Verification items for the finished model (mm, model axes). Round coordinates to 2 decimals unless told otherwise and drop trailing zeros. Write each loop counter-clockwise with the first axis right and the second up, starting at its lowest first coordinate (ties: lowest second). Pieces come first, ordered by that corner, then holes. Notation, with made-up numbers: M 86,24 L 95,24 A30 ccw 95,57 Z; hole C 46.5,25 d10. An arc over 180 degrees is marked long. Write each question's results on one line, items separated by ' | '.
from build123d import *

# Parameters (mm, degrees)
SKETCH1_R           = 2.5527
BOSS_EXTRUDE1_DEPTH = 8.89


with BuildPart() as part:
    # Sketch1 → Boss-Extrude1 (new body)
    with BuildSketch(Plane(origin=(0, 0, 0), x_dir=(1, 0, 0), z_dir=(0, 1, 0))):
        with BuildLine():
            Line((-63.5, 46.99), (63.5, 46.99))
            ThreePointArc((63.5, 46.99), (110.49, 0), (63.5, -46.99))
            Line((63.5, -46.99), (-63.5, -46.99))
            ThreePointArc((-63.5, -46.99), (-110.49, 0), (-63.5, 46.99))
        make_face()
        with Locations(Location((-63.5, 40.64, 0), (0, 0, 270))):
            Circle(SKETCH1_R, mode=Mode.SUBTRACT)
        with Locations(Location((-31.75, 40.64, 0), (0, 0, 270))):
            Circle(SKETCH1_R, mode=Mode.SUBTRACT)
        with Locations(Location((0, 40.64, 0), (0, 0, 270))):
            Circle(SKETCH1_R, mode=Mode.SUBTRACT)
        with Locations(Location((31.75, 40.64, 0), (0, 0, 270))):
            Circle(SKETCH1_R, mode=Mode.SUBTRACT)
        with Locations(Location((63.5, 40.64, 0), (0, 0, 270))):
            Circle(SKETCH1_R, mode=Mode.SUBTRACT)
        with Locations(Location((92.236819587, 28.736819587, 0), (0, 0, 270))):
            Circle(SKETCH1_R, mode=Mode.SUBTRACT)
        with Locations(Location((104.14, 0, 0), (0, 0, 270))):
            Circle(SKETCH1_R, mode=Mode.SUBTRACT)
        with Locations(Location((92.236819587, -28.736819587, 0), (0, 0, 270))):
            Circle(SKETCH1_R, mode=Mode.SUBTRACT)
        with Locations(Location((63.5, -40.64, 0), (0, 0, 270))):
            Circle(SKETCH1_R, mode=Mode.SUBTRACT)
        with Locations(Location((-92.236819587, 28.736819587, 0), (0, 0, 270))):
            Circle(SKETCH1_R, mode=Mode.SUBTRACT)
        with Locations(Location((-104.14, 0, 0), (0, 0, 270))):
            Circle(SKETCH1_R, mode=Mode.SUBTRACT)
        with Locations(Location((-92.236819587, -28.736819587, 0), (0, 0, 270))):
            Circle(SKETCH1_R, mode=Mode.SUBTRACT)
        with Locations(Location((-63.5, -40.64, 0), (0, 0, 270))):
            Circle(SKETCH1_R, mode=Mode.SUBTRACT)
        with Locations(Location((31.75, -40.64, 0), (0, 0, 270))):
            Circle(SKETCH1_R, mode=Mode.SUBTRACT)
        with Locations(Location((0, -40.64, 0), (0, 0, 270))):
            Circle(SKETCH1_R, mode=Mode.SUBTRACT)
        with Locations(Location((-31.75, -40.64, 0), (0, 0, 270))):
            Circle(SKETCH1_R, mode=Mode.SUBTRACT)
    extrude(amount=BOSS_EXTRUDE1_DEPTH)


solid = part.part
1) Sectioned sample at B-B, the plane z = 40.64. Record the cut outline in (x, y).
Calculated:
outline: M -87.09,0 L -66.05,0 L -66.05,8.89 L -87.09,8.89 Z; M -60.95,0 L -34.3,0 L -34.3,8.89 L -60.95,8.89 Z; M -29.2,0 L -2.55,0 L -2.55,8.89 L -29.2,8.89 Z; M 2.55,0 L 29.2,0 L 29.2,8.89 L 2.55,8.89 Z; M 34.3,0 L 60.95,0 L 60.95,8.89 L 34.3,8.89 Z; M 66.05,0 L 87.09,0 L 87.09,8.89 L 66.05,8.89 Z
2) Draft check along X on faces 1 (the cylindrical face through (-110.48, 4.38, 1.03)), 2 (the cylindrical face through (61.95, 4.38, -42.67)), 3 (the flat face through (2, 0, -1)). Enter one of: pulls with the +X half, pulls with the -X half, needs draft (parallel to the pull), parting line crosses it, or undercut.
Calculated:
face 1: pulls with the -X half | face 2: undercut | face 3: needs draft
3) Sectioned sample at C-C, the plane x = -104.14. Record the cut outline in (y, z), and give its area (3 significant figures).
Calculated:
outline: M 0,-23.59 L 8.89,-23.59 L 8.89,-2.55 L 0,-2.55 Z; M 0,2.55 L 8.89,2.55 L 8.89,23.59 L 0,23.59 Z | area: 374 mm²
4) Sectioned sample at A-A, the plane x = 0. Record the cut outline in (y, z).
Calculated:
outline: M 0,-46.99 L 8.89,-46.99 L 8.89,-43.19 L 0,-43.19 Z; M 0,-38.09 L 8.89,-38.09 L 8.89,38.09 L 0,38.09 Z; M 0,43.19 L 8.89,43.19 L 8.89,46.99 L 0,46.99 Z
5) Material ranges on line 1 (Z direction, x = -32, y = 5.5); line 2 (X direction, y = 2, z = -2); line 3 (X direction, y = 7.25, z = -28), recorded low to high. Write a range as [from, to].
Calculated:
line 1: z = [-46.99, -43.18], [-38.1, 38.1], [43.18, 46.99] | line 2: x = [-110.45, -105.73], [-102.55, 102.55], [105.73, 110.45] | line 3: x = [-101.24, -94.68], [-89.79, 89.79], [94.68, 101.24]
6) Sectioned sample at D-D, the plane y = 1.5. Count the separate pieces of the cut face and the enclosed holes in it, and give its area (3 significant figures).
Calculated:
separate pieces: 1 | enclosed holes: 16 | area: 18,500 mm²
7) Depth check by flat-ended pin: P1, Ø5, axis at y = 4.5, z = -4, coming from the -X side; P2, Ø5, axis at x = 76.5, y = 1, coming from the +Z side; P3, Ø1, axis at y = 7.5, z = 31, coming from the +X side. Enter the tip coordinate at first touch or a pass-through.
Calculated:
P1: stops at x = -110.47 | P2: stops at z = 45.8 | P3: stops at x = 99.25
